from build123d import *

# Parameters (mm, degrees)
SKETCH1_W           = 2
SKETCH1_H           = 56
SKETCH1_W_2         = 116
SKETCH1_H_2         = 2
BOSS_EXTRUDE8_DEPTH = 2
FILLET1_R           = 5


with BuildPart() as part:
    # Sketch1 → Boss-Extrude8 (new body)
    with BuildSketch(Plane(origin=(0, 0, 0), x_dir=(1, 0, 0), z_dir=(0, 1, 0))):
        with Locations((-69, 0)):
            Rectangle(SKETCH1_W, SKETCH1_H)
        Polygon((-58, 38), (-58, 40), (-60, 40), (-60, 30), (-70, 30), (-70, 28), (-68, 28), (-58, 28), align=None)
        with Locations((0, 39)):
            Rectangle(SKETCH1_W_2, SKETCH1_H_2)
        Polygon((68, -28), (68, 28), (58, 28), (58, 38), (-58, 38), (-58, 28), (-68, 28), (-68, -28), (-58, -28), (-58, -38), (58, -38), (58, -28), align=None)
        Polygon((70, 28), (70, 30), (60, 30), (60, 40), (58, 40), (58, 38), (58, 28), (68, 28), align=None)
        with Locations((69, 0)):
            Rectangle(SKETCH1_W, SKETCH1_H)
        Polygon((70, -30), (70, -28), (68, -28), (58, -28), (58, -38), (58, -40), (60, -40), (60, -30), align=None)
        with Locations((0, -39)):
            Rectangle(SKETCH1_W_2, SKETCH1_H_2)
        Polygon((-58, -40), (-58, -38), (-58, -28), (-68, -28), (-70, -28), (-70, -30), (-60, -30), (-60, -40), align=None)
    extrude(amount=BOSS_EXTRUDE8_DEPTH)

    # Fillet1
    fillet1_edges = [part.edges().sort_by_distance(p)[0] for p in [
        (60, 1, 30),
        (-60, 1, 30),
        (-60, 1, -30),
        (60, 1, -30),
    ]]
    fillet(fillet1_edges, radius=FILLET1_R)


solid = part.part
Part model, mm, in its own coordinate system. Coordinates: 2 decimals unless noted, no trailing zeros. Write each loop counter-clockwise with the first axis right and the second up, starting at its lowest first coordinate (ties: lowest second). Pieces come first, ordered by that corner, then holes. Notation, with made-up numbers: M 14.25,21 L 61.25,21 A19 cw 61.25,42 Z; hole C -26,82 d11. An arc over 180 degrees is marked long. Return JSON: item names as keys, results as strings.
1. Saw through at B-B, the plane z = -32. Write the cut outline in (x, y), then the cut area to 3 significant figures.
Determined:
{"outline": "M -61,0 L 61,0 L 61,2 L -61,2 Z", "area": "244 mm²"}
2. Flat gauge pins, fed straight in: pin 1 Ø1 at (x, y) = (-68, 1.5) entering from +Z; pin 2 Ø1 at (y, z) = (1, 38) entering from -X; pin 3 Ø6 at (x, z) = (-43.5, -22.5) entering from -Y; pin 4 Ø0.6 at (x, y) = (67.5, 1.5) entering from -Z. Where does each tip first touch, or does it go through?
Determined:
{"pin 1": "z = 30", "pin 2": "x = -60", "pin 3": "y = 0", "pin 4": "z = -30"}
3. Saw through at A-A, the plane y = 0.8. Write the cut outline in (x, z).
Determined:
{"outline": "M -70,-30 L -65,-30 A5 cw -60,-35 L -60,-40 L 60,-40 L 60,-35 A5 cw 65,-30 L 70,-30 L 70,30 L 65,30 A5 cw 60,35 L 60,40 L -60,40 L -60,35 A5 cw -65,30 L -70,30 Z"}
